```python
from build123d import *

# Parameters (mm, degrees)
F0_W      = 93.98
F0_H      = 219.71
F1_DEPTH  = 19.685
F1_FACE_W = 93.98
F1_FACE_H = 219.71
F2_DEPTH  = 19.685
F3_W      = 13.97
F3_H      = 137.16
F3_W_2    = 59.69
F3_H_2    = 20.32
F3_W_3    = 66.04
F3_H_3    = 11.43
F4_DEPTH  = 25.4
F5_DEPTH  = 6.35
F6_W      = 13.97
F6_H      = 137.16
F7_DEPTH  = 7.62
F8_DEPTH  = 12.7
F9_W      = 13.97
F9_H      = 25.4
F10_DEPTH = 5.08
F8_FACE_W = 13.97
F8_FACE_H = 25.4
F11_DEPTH = 5.08


with BuildPart() as f1:
    # F0 (on Top) → F1 (new body)
    with BuildSketch(Plane.XY):
        Rectangle(F0_W, F0_H)
    extrude(amount=F1_DEPTH)

    # F1_face (on face) → F2 (join)
    with BuildSketch(Plane(origin=(0, 0, 0), x_dir=(1, 0, 0), z_dir=(0, 0, -1))):
        Rectangle(F1_FACE_W, F1_FACE_H)
    extrude(amount=F2_DEPTH)

    # F3 (on face) → F4 (cut)
    with BuildSketch(Plane.XY.offset(19.685)):
        Polygon((-34.29, -97.155), (-34.29, -109.855), (-20.32, -109.855), (-20.32, 27.305), (-34.29, 27.305), align=None)
        Polygon((20.32, -109.855), (34.29, -109.855), (34.29, -97.155), (34.29, 27.305), (20.32, 27.305), align=None)
        with Locations((0.635, -41.275)):
            Rectangle(F3_W, F3_H)
        with Locations((-4.445, 50.165)):
            Rectangle(F3_W_2, F3_H_2)
        with Locations((-1.27, 78.74)):
            Rectangle(F3_W_3, F3_H_3)
    extrude(amount=-F4_DEPTH, mode=Mode.SUBTRACT)

    # F3 (on face) → F5 (cut)
    with BuildSketch(Plane.XY.offset(19.685)):
        with Locations((-4.445, 50.165)):
            Rectangle(F3_W_2, F3_H_2)
    extrude(amount=-F5_DEPTH, mode=Mode.SUBTRACT)

    # F6 (on face) → F7 (join)
    with BuildSketch(Plane.XY.offset(19.685)):
        with Locations((-27.305, -41.275)):
            Rectangle(F6_W, F6_H)
        with Locations((0.635, -41.275)):
            Rectangle(F6_W, F6_H)
        with Locations((27.305, -41.275)):
            Rectangle(F6_W, F6_H)
    extrude(amount=-F7_DEPTH)

    # F3 (on face) → F8 (cut)
    with BuildSketch(Plane.XY.offset(19.685)):
        Polygon((20.32, -109.855), (34.29, -109.855), (34.29, -97.155), (34.29, 27.305), (20.32, 27.305), align=None)
        with Locations((0.635, -41.275)):
            Rectangle(F3_W, F3_H)
        Polygon((-34.29, -97.155), (-34.29, -109.855), (-20.32, -109.855), (-20.32, 27.305), (-34.29, 27.305), align=None)
    extrude(amount=-F8_DEPTH, mode=Mode.SUBTRACT)

    # F9 (on face) → F10 (join)
    with BuildSketch(Plane.XZ.offset(109.855)):
        with Locations((-27.305, 6.985)):
            Rectangle(F9_W, F9_H)
        with Locations((0.635, 6.985)):
            Rectangle(F9_W, F9_H)
        with Locations((27.305, 6.985)):
            Rectangle(F9_W, F9_H)
    extrude(amount=-F10_DEPTH)

    # F8_face (on face) → F11 (cut)
    with BuildSketch(Plane(origin=(-27.305, 27.305, 6.985), x_dir=(1, 0, 0), z_dir=(0, -1, 0))):
        Rectangle(F8_FACE_W, F8_FACE_H)
        with Locations((27.94, 0)):
            Rectangle(F8_FACE_W, F8_FACE_H)
        with Locations((54.61, 0)):
            Rectangle(F8_FACE_W, F8_FACE_H)
    extrude(amount=-F11_DEPTH, mode=Mode.SUBTRACT)


solid = f1.part
```
For this review, take the finished solid that the model builds, in its own axes (mm). A direction names the side the tool comes from. Round coordinates to 2 decimals unless told otherwise and drop trailing zeros. Write each loop counter-clockwise with the first axis right and the second up, starting at its lowest first coordinate (ties: lowest second). Pieces come first, ordered by that corner, then holes. Notation, with made-up numbers: (42.5, -6.75) - (73.5, -6.75) arc R19 ccw to (73.5, 21.25) - close; hole circle Ø10 at (7, 2.25). An arc over 180 degrees is marked (long way). Put each result on its own line as item: value.
Q1. We need section D-D (x = -18). Give the boundary of the cut face in (y, z) (3 decimals).
Solved:
outline: (-109.855, -19.685) - (109.855, -19.685) - (109.855, 19.685) - (84.455, 19.685) - (84.455, -5.715) - (73.025, -5.715) - (73.025, 19.685) - (60.325, 19.685) - (60.325, -5.715) - (40.005, -5.715) - (40.005, 19.685) - (-109.855, 19.685) - close
Q2. We need section C-C (y = -22). Give the boundary of the cut face in (x, z) (3 decimals), and give its area (3 significant figures).
Solved:
outline: (-46.99, -19.685) - (46.99, -19.685) - (46.99, 19.685) - (34.29, 19.685) - (34.29, -5.715) - (20.32, -5.715) - (20.32, 19.685) - (7.62, 19.685) - (7.62, -5.715) - (-6.35, -5.715) - (-6.35, 19.685) - (-20.32, 19.685) - (-20.32, -5.715) - (-34.29, -5.715) - (-34.29, 19.685) - (-46.99, 19.685) - close
area: 2,640 mm2
Q3. Mouldability with a two-part tool opening along X and no side actions: class faces 3 (the face through (-1, -109.855, 0)), 4 (the face through (46.99, 2, 0)), 5 (the face through (-27, 32.385, 7)) as released by +X, released by -X, zero draft, split by the parting line, or undercut.
Solved:
face 3: zero draft
face 4: released by +X
face 5: undercut
Q4. Machinability: for faces 1 (the face through (-20.32, -37, 7)), 2 (the face through (10, -2, 19.685)), which of the approach directions +Z, -Z, +X, -X, +Y, -Y give a long, thin tool a straight path to every point of the face, cutting with its end or side? Answer none if there is none.
Solved:
face 1: +Z
face 2: +Z, +X, -X, +Y, -Y
Q5. We need section A-A (z = 7.5). Give the boundary of the cut face in (x, y) (3 decimals), and give its area (3 significant figures).
Solved:
outline: (-46.99, -109.855) - (46.99, -109.855) - (46.99, 109.855) - (-46.99, 109.855) - close; hole (-34.29, -104.775) - (-20.32, -104.775) - (-20.32, 32.385) - (-34.29, 32.385) - close; hole (-34.29, 40.005) - (25.4, 40.005) - (25.4, 60.325) - (-34.29, 60.325) - close; hole (-34.29, 73.025) - (31.75, 73.025) - (31.75, 84.455) - (-34.29, 84.455) - close; hole (-6.35, -104.775) - (7.62, -104.775) - (7.62, 32.385) - (-6.35, 32.385) - close; hole (20.32, -104.775) - (34.29, -104.775) - (34.29, 32.385) - (20.32, 32.385) - close
area: 12,900 mm2
Q6. We need section B-B (x = 0). Give the boundary of the cut face in (y, z) (3 decimals), and give its area (3 significant figures).
Solved:
outline: (-109.855, -19.685) - (109.855, -19.685) - (109.855, 19.685) - (84.455, 19.685) - (84.455, -5.715) - (73.025, -5.715) - (73.025, 19.685) - (60.325, 19.685) - (60.325, -5.715) - (40.005, -5.715) - (40.005, 19.685) - (32.385, 19.685) - (32.385, -5.715) - (-104.775, -5.715) - (-104.775, 19.685) - (-109.855, 19.685) - close
area: 4,360 mm2
Q7. Wall thickness on probe 1 along Y at (x, z) = (-25, 7) (3 decimals); probe 2 along Y at (x, z) = (-7.5, 10.5) (3 decimals); probe 3 along X at (y, z) = (-33, 17): over which ranges is each line inside the solid? List them lowest first.
Solved:
probe 1: y = -109.855 to -104.775, 32.385 to 40.005, 60.325 to 73.025, 84.455 to 109.855
probe 2: y = -109.855 to 40.005, 60.325 to 73.025, 84.455 to 109.855
probe 3: x = -46.99 to -34.29, -20.32 to -6.35, 7.62 to 20.32, 34.29 to 46.99
Q8. Insertion check: pin 1 Ø7 at (x, y) = (30, -64.5) entering from +Z (3 decimals). The pin has a flat end and moves straight along its axis. Give the tip position at first contact, or say it passes through.
Solved:
pin 1: stops at z = -5.715
